Verification items for the finished model (mm, model axes). A direction names the side the tool comes from. Coordinates: 2 decimals unless noted, no trailing zeros. Loops run counter-clockwise (first coordinate to the right, second up) from the corner with the lowest first, then second, coordinate; pieces in that order, holes last. Notation, with made-up numbers: (76.25, 32) -> (93.25, 32) arc R15 cw to (93.25, 46) -> close; hole circle Ø3 at (-23.75, 5). An arc over 180 degrees is marked (long way). Write item = value, one per line.
```python
from build123d import *

# Parameters (mm, degrees)
SKETCH1_R           = 1.75
BOSS_EXTRUDE1_DEPTH = 4
SKETCH2_W           = 5
SKETCH2_H           = 38
CUT_EXTRUDE1_DEPTH  = 145.364122967
SKETCH3_W           = 8
SKETCH3_H           = 76.5
BOSS_EXTRUDE2_DEPTH = 5
FILLET1_R           = 2
SKETCH4_R           = 1.75
CUT_EXTRUDE2_DEPTH  = 145.395290782


with BuildPart() as part:
    # Sketch1 → Boss-Extrude1 (new body)
    with BuildSketch(Plane.XY):
        with BuildLine():
            Line((-35, 140), (-28, 140))
            ThreePointArc((-28, 140), (0, 112), (28, 140))
            Line((28, 140), (35, 140))
            Line((35, 140), (35, 0))
            Line((35, 0), (-35, 0))
            Line((-35, 0), (-35, 140))
        make_face()
        with Locations((-25, 60)):
            Circle(SKETCH1_R, mode=Mode.SUBTRACT)
        with Locations((25, 60)):
            Circle(SKETCH1_R, mode=Mode.SUBTRACT)
        with Locations((-10, 10)):
            Circle(SKETCH1_R, mode=Mode.SUBTRACT)
        with Locations((10, 10)):
            Circle(SKETCH1_R, mode=Mode.SUBTRACT)
        with Locations((-10, 20)):
            Circle(SKETCH1_R, mode=Mode.SUBTRACT)
        with Locations((10, 20)):
            Circle(SKETCH1_R, mode=Mode.SUBTRACT)
        with Locations((-10, 30)):
            Circle(SKETCH1_R, mode=Mode.SUBTRACT)
        with Locations((10, 30)):
            Circle(SKETCH1_R, mode=Mode.SUBTRACT)
    extrude(amount=BOSS_EXTRUDE1_DEPTH)

    # Sketch2 → Cut-Extrude1 (cut, through all)
    with BuildSketch(Plane(origin=(0, 0, 0), x_dir=(-1, 0, 0), z_dir=(0, 0, -1))):
        with Locations((0, 121)):
            Rectangle(SKETCH2_W, SKETCH2_H)
    extrude(amount=-CUT_EXTRUDE1_DEPTH, mode=Mode.SUBTRACT)

    # Sketch3 → Boss-Extrude2 (add)
    with BuildSketch(Plane(origin=(0, 0, 0), x_dir=(-1, 0, 0), z_dir=(0, 0, -1))):
        with Locations((0, 58.75)):
            Rectangle(SKETCH3_W, SKETCH3_H)
    extrude(amount=BOSS_EXTRUDE2_DEPTH)

    # Fillet1
    fillet1_edges = [part.edges().sort_by_distance(p)[0] for p in [
        (4, 58.75, -5),
        (-4, 58.75, -5),
    ]]
    fillet(fillet1_edges, radius=FILLET1_R)

    # Sketch4 → Cut-Extrude2 (cut, through all)
    with BuildSketch(Plane(origin=(0, 0, 0), x_dir=(-1, 0, 0), z_dir=(0, 0, -1))):
        with Locations((-25, 90)):
            Circle(SKETCH4_R)
        with Locations((25, 90)):
            Circle(SKETCH4_R)
    extrude(amount=-CUT_EXTRUDE2_DEPTH, mode=Mode.SUBTRACT)


solid = part.part
```
1) Sectioned sample at B-B, the plane x = -25. Record the cut outline in (y, z), plus the area to 3 significant figures.
Ans:
outline = (0, 0) -> (58.25, 0) -> (58.25, 4) -> (0, 4) -> close; (61.75, 0) -> (88.25, 0) -> (88.25, 4) -> (61.75, 4) -> close; (91.75, 0) -> (127.39, 0) -> (127.39, 4) -> (91.75, 4) -> close
area = 482 mm2
2) Tool access check on faces 1 (the face through (0, 102, 2)), 2 (the face through (4, 58, -1)), 3 (the face through (0, 97, -2)). Record the directions out of +Z, -Z, +X, -X, +Y, -Y that give a thin tool (end or side, any length) a straight path to the whole face; none if there is none.
Ans:
face_1 = +Z, -Z, +Y
face_2 = -Z, +X, +Y, -Y
face_3 = -Z, +X, -X, +Y
3) Depth check by flat-ended pin: pin 1 Ø3 at (x, y) = (-10, 10) entering from +Z; pin 2 Ø4.5 at (x, z) = (0, 2.5) entering from +Y; pin 3 Ø4.5 at (x, y) = (-25, 90) entering from -Z; pin 4 Ø1.5 at (y, z) = (53, -2) entering from +X. Enter the tip coordinate at first touch or a pass-through.
Ans:
pin_1 = through
pin_2 = 102
pin_3 = 0
pin_4 = 4
4) Sectioned sample at D-D, the plane y = 10. Record the cut outline in (x, z), plus the area to 3 significant figures.
Ans:
outline = (-35, 0) -> (-11.75, 0) -> (-11.75, 4) -> (-35, 4) -> close; (-8.25, 0) -> (8.25, 0) -> (8.25, 4) -> (-8.25, 4) -> close; (11.75, 0) -> (35, 0) -> (35, 4) -> (11.75, 4) -> close
area = 252 mm2
5) Material ranges on line 1 (Y direction, x = -10, z = 0.85); line 2 (Z direction, x = -6, y = 107); line 3 (Y direction, x = 25, z = 2.85), recorded low to high.
Ans:
line_1 = 0 to 8.25, 11.75 to 18.25, 21.75 to 28.25, 31.75 to 113.85
line_2 = 0 to 4
line_3 = 0 to 58.25, 61.75 to 88.25, 91.75 to 127.39
6) Release check for a two-part mould opening along Y. For faces 4 (the face through (10.9, 11.5, 2)), 5 (the face through (20.467, 120.892, 1.972)), 6 (the face through (0, 59, -5)), 7 (the face through (11.669, 30.526, 1.972)) record: pulls with the +Y half, pulls with the -Y half, needs draft (parallel to the pull), parting line crosses it, or undercut.
Ans:
face_4 = undercut
face_5 = pulls with the +Y half
face_6 = needs draft
face_7 = undercut
7) Sectioned sample at A-A, the plane y = 90. Record the cut outline in (x, z), plus the area to 3 significant figures.
Ans:
outline = (-35, 0) -> (-26.75, 0) -> (-26.75, 4) -> (-35, 4) -> close; (-23.25, 0) -> (-4, 0) -> (-4, -3) arc R2 ccw to (-2, -5) -> (2, -5) arc R2 ccw to (4, -3) -> (4, 0) -> (23.25, 0) -> (23.25, 4) -> (-23.25, 4) -> close; (26.75, 0) -> (35, 0) -> (35, 4) -> (26.75, 4) -> close
area = 290 mm2
8) Sectioned sample at C-C, the plane x = 10. Record the cut outline in (y, z).
Ans:
outline = (0, 0) -> (8.25, 0) -> (8.25, 4) -> (0, 4) -> close; (11.75, 0) -> (18.25, 0) -> (18.25, 4) -> (11.75, 4) -> close; (21.75, 0) -> (28.25, 0) -> (28.25, 4) -> (21.75, 4) -> close; (31.75, 0) -> (113.85, 0) -> (113.85, 4) -> (31.75, 4) -> close
